from build123d import *

# Parameters (mm, degrees)
SKETCH2_W           = 20.45
SKETCH2_H           = 19
BOSS_EXTRUDE1_DEPTH = 7
SKETCH3_W           = 18.45
SKETCH3_H           = 17.2
CUT_EXTRUDE1_DEPTH  = 5
SKETCH7_R           = 1.65
CUT_EXTRUDE2_DEPTH  = 2
SKETCH13_W          = 16
SKETCH13_H          = 2
CUT_EXTRUDE4_DEPTH  = 2
SKETCH15_W          = 20.45
SKETCH15_H          = 0.9
BOSS_EXTRUDE2_DEPTH = 5
SKETCH16_R          = 1.15
CUT_EXTRUDE5_DEPTH  = 0.9
FILLET2_R           = 0.25


with BuildPart() as part:
    # Sketch2 → Boss-Extrude1 (new body)
    with BuildSketch(Plane(origin=(0, 0, 0), x_dir=(1, 0, 0), z_dir=(0, 1, 0))):
        Rectangle(SKETCH2_W, SKETCH2_H)
    extrude(amount=BOSS_EXTRUDE1_DEPTH)

    # Sketch3 → Cut-Extrude1 (cut)
    with BuildSketch(Plane(origin=(0, 7, 0), x_dir=(1, 0, 0), z_dir=(0, 1, 0))):
        Rectangle(SKETCH3_W, SKETCH3_H)
    extrude(amount=-CUT_EXTRUDE1_DEPTH, mode=Mode.SUBTRACT)

    # Sketch7 → Cut-Extrude2 (cut)
    with BuildSketch(Plane(origin=(0, 2, 0), x_dir=(1, 0, 0), z_dir=(0, 1, 0))):
        with Locations(Location((-5.495, 5, 0), (0, 0, 270))):
            Circle(SKETCH7_R)
        with Locations(Location((5.505, 5, 0), (0, 0, 270))):
            Circle(SKETCH7_R)
    extrude(amount=-CUT_EXTRUDE2_DEPTH, mode=Mode.SUBTRACT)

    # Sketch13 → Cut-Extrude4 (cut)
    with BuildSketch(Plane(origin=(0, 2, 0), x_dir=(1, 0, 0), z_dir=(0, 1, 0))):
        with Locations((0, -5)):
            Rectangle(SKETCH13_W, SKETCH13_H)
    extrude(amount=-CUT_EXTRUDE4_DEPTH, mode=Mode.SUBTRACT)

    # Sketch15 → Boss-Extrude2 (add)
    with BuildSketch(Plane(origin=(0, 7, 0), x_dir=(1, 0, 0), z_dir=(0, 1, 0))):
        with Locations((0, 9.05)):
            Rectangle(SKETCH15_W, SKETCH15_H)
    extrude(amount=BOSS_EXTRUDE2_DEPTH)

    # Sketch16 → Cut-Extrude5 (cut)
    with BuildSketch(Plane.XY.offset(-8.6)):
        with Locations((0, 9.5)):
            Circle(SKETCH16_R)
    extrude(amount=-CUT_EXTRUDE5_DEPTH, mode=Mode.SUBTRACT)

    # Fillet2
    fillet2_edges = [part.edges().sort_by_distance(p)[0] for p in [
        (10.225, 7, 0.45),
        (0, 0, -9.5),
        (-10.225, 7, 0.45),
        (10.225, 0, 0),
        (-10.225, 12, -9.05),
        (0, 12, -8.6),
        (10.225, 12, -9.05),
        (0, 0, 9.5),
        (0, 12, -9.5),
        (-10.225, 0, 0),
        (-10.225, 6, -9.5),
        (10.225, 6, -9.5),
        (10.225, 3.5, 9.5),
        (-10.225, 3.5, 9.5),
        (0, 7, 9.5),
    ]]
    fillet(fillet2_edges, radius=FILLET2_R)


solid = part.part
Can you work these out from the model? Positions are in its coordinate system, mm. A direction names the side the tool comes from. Round coordinates to 2 decimals unless told otherwise and drop trailing zeros. Order: outer loops, then holes, each group sorted by start corner. A loop starts at its lowest first (then second) coordinate and runs counter-clockwise, first axis right, second up. Notation, with made-up numbers: (-2, 11.5) -> (20, 11.5) arc R21 ccw to (20, 36.5) -> close; hole circle Ø7 at (-40, 35.5). An arc over 180 degrees is marked (long way). Write each question's results on one line, items separated by ' | '. Start each with the question number.
Item 1: Will this pin go through, and if not, where does the flat tip stop? pin 1 (1 mm diameter, centred on x = -7, z = 6.5, fed in from +Y).
Item 2: If we section it at D-D, the plane y = 5: Write out the boundary of the cut face in (x, z) (3 decimals).
Item 3: If we section it at A-A, the plane y = 9.5: Write out the boundary of the cut face in (x, z) (3 decimals), then the cut area to 3 significant figures.
Item 4: Thinking about a two-plate mould opening in Z: for faces 1 (the flat face through (0, 6, -9.5)), 2 (the flat face through (0, 7, 9)), 3 (the flat face through (-8, 1, 5)), which applies, +Z half, -Z half, draft (parallel to the pull), parting line (faces both ways), or undercut?
Item 5: If we section it at C-C, the plane x = -2.5: Write out the boundary of the cut face in (y, z), then the cut area to 3 significant figures.
Item 6: Which directions (+Z, -Z, +X, -X, +Y, -Y) give clear straight access to the entire face, cutting with the end or side of a thin tool? Please do faces 4 (the flat face through (0, 0, 0)), 5 (the flat face through (0, 2, 0)), 6 (the flat face through (0, 1, 6)).
Item 7: Please list where these lines run through material, in increasing order: L1, parallel to X at y = 1.55, z = -5 (3 decimals); L2, parallel to Z at x = 2.75, y = 4.75; L3, parallel to Z at x = -2.75, y = 1.5.
Item 8: If we section it at B-B, the plane z = -5: Write out the boundary of the cut face in (x, y) (3 decimals).
Results:
1) pin 1: stops at y = 2
2) outline: (-10.225, -9.25) arc R0.25 ccw to (-9.975, -9.5) -> (9.975, -9.5) arc R0.25 ccw to (10.225, -9.25) -> (10.225, 9.25) arc R0.25 ccw to (9.975, 9.5) -> (-9.975, 9.5) arc R0.25 ccw to (-10.225, 9.25) -> close; hole (-9.225, -8.6) -> (9.225, -8.6) -> (9.225, 8.6) -> (-9.225, 8.6) -> close
3) outline: (-10.225, -9.25) arc R0.25 ccw to (-9.975, -9.5) -> (-1.15, -9.5) -> (-1.15, -8.6) -> (-10.225, -8.6) -> close; (1.15, -9.5) -> (9.975, -9.5) arc R0.25 ccw to (10.225, -9.25) -> (10.225, -8.6) -> (1.15, -8.6) -> close | area: 16.3 mm2
4) face 1: -Z half | face 2: draft | face 3: undercut
5) outline: (0, -9.25) arc R0.25 ccw to (0.25, -9.5) -> (11.75, -9.5) arc R0.25 ccw to (12, -9.25) -> (12, -8.85) arc R0.25 ccw to (11.75, -8.6) -> (2, -8.6) -> (2, 4) -> (0, 4) -> close; (0, 6) -> (2, 6) -> (2, 8.6) -> (7, 8.6) -> (7, 9.25) arc R0.25 ccw to (6.75, 9.5) -> (0.25, 9.5) arc R0.25 ccw to (0, 9.25) -> close | area: 47.4 mm2
6) face 4: +Z, -Z, +X, -X, -Y | face 5: +Y | face 6: +Y, -Y
7) L1: x = -10.225 to -7.145, -3.845 to 3.855, 7.155 to 10.225 | L2: z = -9.5 to -8.6, 8.6 to 9.5 | L3: z = -9.5 to 4, 6 to 9.5
8) outline: (-10.225, 0.25) arc R0.25 ccw to (-9.975, 0) -> (-7.145, 0) -> (-7.145, 2) -> (-9.225, 2) -> (-9.225, 7) -> (-9.975, 7) arc R0.25 ccw to (-10.225, 6.75) -> close; (-3.845, 0) -> (3.855, 0) -> (3.855, 2) -> (-3.845, 2) -> close; (7.155, 0) -> (9.975, 0) arc R0.25 ccw to (10.225, 0.25) -> (10.225, 6.75) arc R0.25 ccw to (9.975, 7) -> (9.225, 7) -> (9.225, 2) -> (7.155, 2) -> close
